The listing builds one solid part. Answer for the finished solid, in the listing's coordinates (mm). Coordinates: 2 decimals unless noted, no trailing zeros. Order: outer loops, then holes, each group sorted by start corner. A loop starts at its lowest first (then second) coordinate and runs counter-clockwise, first axis right, second up. Notation, with made-up numbers: (-14.5, -6) - (24.5, -6) arc R25 ccw to (24.5, 31) - close; hole circle Ø10 at (56.25, 82). An arc over 180 degrees is marked (long way). Use a Markdown table: item, result. Add a question column.
Item 1: Find the intervals of material crossed by line 1 along X through (y, z) = (27, 1.9); line 2 along Y through (x, z) = (15, 2.2); line 3 along X through (y, z) = (-26, 1.7), in increasing order.
Item 2: The part is cut by section B-B, the plane x = 0. Give the vertices of the cut face in (y, z).
Item 3: A flat-ended cylindrical pin translates along its axis: P1, Ø2.5, axis at x = -30, y = 0, coming from the +Z side. Find the tip coordinate at first contact, or state that the pin passes through.
Item 4: The part is cut by section A-A, the plane x = -12.5. Give the vertices of the cut face in (y, z), then the cut area to 3 significant figures.
Item 5: The part is cut by section D-D, the plane x = 30. Give the vertices of the cut face in (y, z), then the cut area to 3 significant figures.
Item 6: The part is cut by section C-C, the plane z = 1.35. State how many separate pieces and enclosed holes the cut face has, then the cut area to 3 significant figures.
from build123d import *

# Parameters (mm, degrees)
EXTRUDE_1_DEPTH     = 3
SKETCH_2_R          = 10
SKETCH_2_R_2        = 1.5
CUT_EXTRUDE_1_DEPTH = 3
SKETCH_3_R          = 1.5
CUT_EXTRUDE_2_DEPTH = 3
FILLET_1_R          = 5


with BuildPart() as part:
    # 草图1 → 凸台-拉伸1 (new body)
    with BuildSketch(Plane.XY):
        Polygon((34.641016151, 0), (17.320508076, 30), (-17.320508076, 30), (-34.641016151, 0), (-17.320508076, -30), (17.320508076, -30), align=None)
    extrude(amount=EXTRUDE_1_DEPTH)

    # 草图2 → 切除-拉伸1 (cut)
    with BuildSketch(Plane.XY.offset(3)):
        Circle(SKETCH_2_R)
        with Locations((-12.5, 9.5)):
            Circle(SKETCH_2_R_2)
        with Locations((12.5, 9.5)):
            Circle(SKETCH_2_R_2)
        with Locations((-12.5, -9.5)):
            Circle(SKETCH_2_R_2)
        with Locations((12.5, -9.5)):
            Circle(SKETCH_2_R_2)
    extrude(amount=-CUT_EXTRUDE_1_DEPTH, mode=Mode.SUBTRACT)

    # 草图3 → 切除-拉伸2 (cut)
    with BuildSketch(Plane.XY.offset(3)):
        with Locations((-30, 0)):
            Circle(SKETCH_3_R)
        with Locations((30, 0)):
            Circle(SKETCH_3_R)
        with Locations((-14.820508076, -25.669872981)):
            Circle(SKETCH_3_R)
        with Locations((14.820508076, -25.669872981)):
            Circle(SKETCH_3_R)
        with Locations((-14.820508076, 25.669872981)):
            Circle(SKETCH_3_R)
        with Locations((14.820508076, 25.669872981)):
            Circle(SKETCH_3_R)
    extrude(amount=-CUT_EXTRUDE_2_DEPTH, mode=Mode.SUBTRACT)

    # 圆角1
    fillet_1_edges = [part.edges().sort_by_distance(p)[0] for p in [
        (17.320508076, -30, 1.5),
        (-17.320508076, -30, 1.5),
        (-34.641016151, 0, 1.5),
        (-17.320508076, 30, 1.5),
        (17.320508076, 30, 1.5),
        (34.641016151, 0, 1.5),
    ]]
    fillet(fillet_1_edges, radius=FILLET_1_R)


solid = part.part
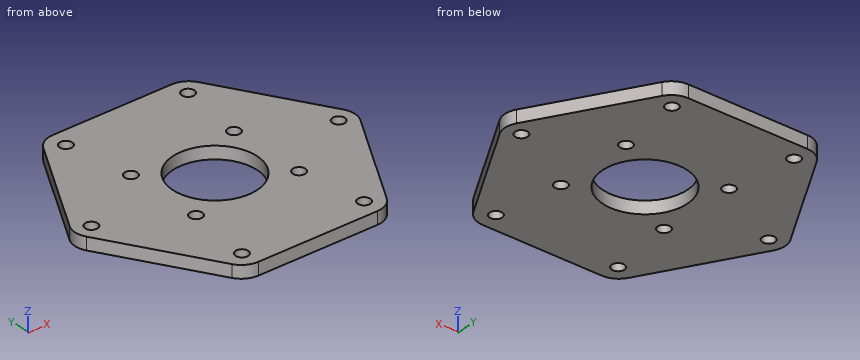
Solution:
| question | item | result |
|---|---|---|
| 1 | line 1 | x = -19.05 to -15.51, -14.13 to 14.13, 15.51 to 19.05 |
| 1 | line 2 | y = -29.97 to -27.16, -24.18 to 24.18, 27.16 to 29.97 |
| 1 | line 3 | x = -19.63 to -16.28, -13.36 to 13.36, 16.28 to 19.63 |
| 2 | outline | (-30, 0) - (-10, 0) - (-10, 3) - (-30, 3) - close; (10, 0) - (30, 0) - (30, 3) - (10, 3) - close |
| 3 | P1 | passes through |
| 4 | outline | (-30, 0) - (-11, 0) - (-11, 3) - (-30, 3) - close; (-8, 0) - (8, 0) - (8, 3) - (-8, 3) - close; (11, 0) - (30, 0) - (30, 3) - (11, 3) - close |
| 4 | area | 162 mm2 |
| 5 | outline | (-8.04, 0) - (-1.5, 0) - (-1.5, 3) - (-8.04, 3) - close; (1.5, 0) - (8.04, 0) - (8.04, 3) - (1.5, 3) - close |
| 5 | area | 39.2 mm2 |
| 6 | separate pieces | 1 |
| 6 | enclosed holes | 11 |
| 6 | area | 2,720 mm2 |
